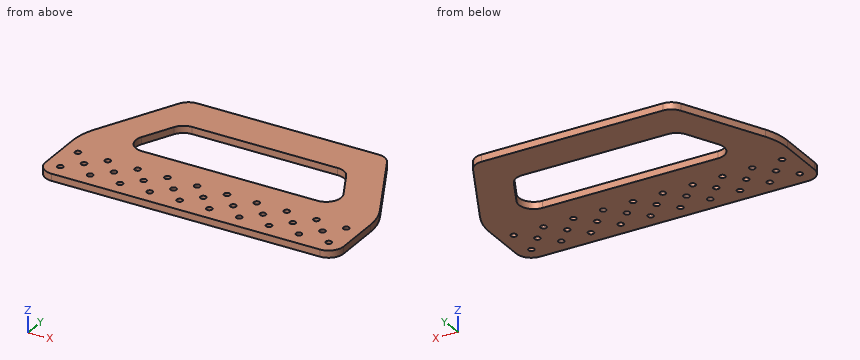
from build123d import *

# Parameters (mm, degrees)
BOSS_EXTRUDE1_DEPTH = 6
SKETCH2_R           = 2.4892
CUT_EXTRUDE1_DEPTH  = 294.692326083


with BuildPart() as part:
    # Sketch1 → Boss-Extrude1 (new body)
    with BuildSketch(Plane.XY):
        with BuildLine():
            Line((12.7, 0), (241.3, 0))
            ThreePointArc((241.3, 0), (250.280256121, 3.719743879), (254, 12.7))
            Line((254, 12.7), (254, 51.507746743))
            ThreePointArc((254, 51.507746743), (252.641048665, 63.179195107), (248.636901303, 74.226197394))
            Line((248.636901303, 74.226197394), (215.600193669, 140.299612663))
            ThreePointArc((215.600193669, 140.299612663), (210.917753467, 145.423265266), (204.240968343, 147.32))
            Line((204.240968343, 147.32), (49.759031657, 147.32))
            ThreePointArc((49.759031657, 147.32), (43.082246533, 145.423265266), (38.399806331, 140.299612663))
            Line((38.399806331, 140.299612663), (5.363098697, 74.226197394))
            ThreePointArc((5.363098697, 74.226197394), (1.358951335, 63.179195107), (0, 51.507746743))
            Line((0, 51.507746743), (0, 12.7))
            ThreePointArc((0, 12.7), (3.719743879, 3.719743879), (12.7, 0))
        make_face()
        with BuildLine():
            Line((40.939806331, 81.879612663), (53.639806331, 107.279612663))
            ThreePointArc((53.639806331, 107.279612663), (58.322246533, 112.403265266), (64.999031657, 114.3))
            Line((64.999031657, 114.3), (189.000968343, 114.3))
            ThreePointArc((189.000968343, 114.3), (195.677753467, 112.403265266), (200.360193669, 107.279612663))
            Line((200.360193669, 107.279612663), (213.060193669, 81.879612663))
            ThreePointArc((213.060193669, 81.879612663), (212.504233609, 69.523214876), (201.700968343, 63.5))
            Line((201.700968343, 63.5), (52.299031657, 63.5))
            ThreePointArc((52.299031657, 63.5), (41.495766391, 69.523214876), (40.939806331, 81.879612663))
        make_face(mode=Mode.SUBTRACT)
    extrude(amount=BOSS_EXTRUDE1_DEPTH)

    # Sketch2 → Cut-Extrude1 (cut, through all)
    with BuildSketch(Plane.XY.offset(6)):
        with Locations((241.3, 12.7)):
            Circle(SKETCH2_R)
        with Locations((215.9, 12.7)):
            Circle(SKETCH2_R)
        with Locations((190.5, 12.7)):
            Circle(SKETCH2_R)
        with Locations((165.1, 12.7)):
            Circle(SKETCH2_R)
        with Locations((139.7, 12.7)):
            Circle(SKETCH2_R)
        with Locations((114.3, 12.7)):
            Circle(SKETCH2_R)
        with Locations((88.9, 12.7)):
            Circle(SKETCH2_R)
        with Locations((63.5, 12.7)):
            Circle(SKETCH2_R)
        with Locations((38.1, 12.7)):
            Circle(SKETCH2_R)
        with Locations((12.7, 12.7)):
            Circle(SKETCH2_R)
        with Locations((215.9, 38.1)):
            Circle(SKETCH2_R)
        with Locations((190.5, 38.1)):
            Circle(SKETCH2_R)
        with Locations((165.1, 38.1)):
            Circle(SKETCH2_R)
        with Locations((139.7, 38.1)):
            Circle(SKETCH2_R)
        with Locations((114.3, 38.1)):
            Circle(SKETCH2_R)
        with Locations((88.9, 38.1)):
            Circle(SKETCH2_R)
        with Locations((63.5, 38.1)):
            Circle(SKETCH2_R)
        with Locations((38.1, 38.1)):
            Circle(SKETCH2_R)
        with Locations((12.7, 38.1)):
            Circle(SKETCH2_R)
        with Locations((241.3, 38.1)):
            Circle(SKETCH2_R)
        with Locations((25.4, 25.4)):
            Circle(SKETCH2_R)
        with Locations((50.8, 25.4)):
            Circle(SKETCH2_R)
        with Locations((76.2, 25.4)):
            Circle(SKETCH2_R)
        with Locations((101.6, 25.4)):
            Circle(SKETCH2_R)
        with Locations((127, 25.4)):
            Circle(SKETCH2_R)
        with Locations((152.4, 25.4)):
            Circle(SKETCH2_R)
        with Locations((177.8, 25.4)):
            Circle(SKETCH2_R)
        with Locations((203.2, 25.4)):
            Circle(SKETCH2_R)
        with Locations((228.6, 25.4)):
            Circle(SKETCH2_R)
    extrude(amount=-CUT_EXTRUDE1_DEPTH, mode=Mode.SUBTRACT)


solid = part.part
Read the model definition and answer for the solid it produces. Units are mm, in the model's axes. Give positions to 0.01 mm unless a question says otherwise; leave off trailing zeros. Loops run counter-clockwise (first coordinate to the right, second up) from the corner with the lowest first, then second, coordinate; pieces in that order, holes last. Notation, with made-up numbers: (15, 44.25) - (72, 44.25) arc R19 cw to (72, 49.25) - close; hole circle Ø2 at (-34, 27.25). An arc over 180 degrees is marked (long way). Answer as CSV lines item,"result". Start each with the question number.
1) Find section B-B (y = 69). Write down the section's boundary in (x, z).
2) Find section A-A (x = 71). Write down the section's boundary in (y, z), then the cut area to 3 significant figures.
3) This flat-tipped pin is pushed along its axis until it touches: pin 1 Ø1.5 at (y, z) = (101, 1.5) entering from +X (3 decimals). Where does it stop, or does it pass through?
4) Find section D-D (y = 38.1). State how many separate pieces and enclosed holes the cut face has, then the cut area to 3 significant figures.
5) Find section C-C (x = 139.7). Write down the section's boundary in (y, z), then the cut area to 3 significant figures.
6) Straight lines are drawn through the part: L1, parallel to Y at x = 152, z = 3.6; L2, parallel to Y at x = 88.9, z = 3.35; L3, parallel to Y at x = 67, z = 4. For each, find the intervals that lie inside material, in ascending order. Write a range as from..to.
Findings below:
1,outline,"(3.11, 0) - (41.84, 0) - (41.84, 6) - (3.11, 6) - close; (212.16, 0) - (250.89, 0) - (250.89, 6) - (212.16, 6) - close"
2,outline,"(0, 0) - (63.5, 0) - (63.5, 6) - (0, 6) - close; (114.3, 0) - (147.32, 0) - (147.32, 6) - (114.3, 6) - close"
2,area,"579 mm^2"
3,pin 1,"x = 235.625"
4,separate pieces,"11"
4,enclosed holes,"0"
4,area,"1,230 mm^2"
5,outline,"(0, 0) - (10.21, 0) - (10.21, 6) - (0, 6) - close; (15.19, 0) - (35.61, 0) - (35.61, 6) - (15.19, 6) - close; (40.59, 0) - (63.5, 0) - (63.5, 6) - (40.59, 6) - close; (114.3, 0) - (147.32, 0) - (147.32, 6) - (114.3, 6) - close"
5,area,"519 mm^2"
6,L1,"0..22.94, 27.86..63.5, 114.3..147.32"
6,L2,"0..10.21, 15.19..35.61, 40.59..63.5, 114.3..147.32"
6,L3,"0..63.5, 114.3..147.32"
